Work out the finished part from the listing and answer in its coordinate system (mm). A direction names the side the tool comes from. Coordinates: 2 decimals unless noted, no trailing zeros. Order: outer loops, then holes, each group sorted by start corner. A loop starts at its lowest first (then second) coordinate and runs counter-clockwise, first axis right, second up. Notation, with made-up numbers: (33, 76.5) - (47, 76.5) arc R18 cw to (47, 80.5) - close; hole circle Ø10 at (47, 4.25). An arc over 180 degrees is marked (long way). Answer as a JSON object with one key per item and string values. Group by question number.
1) Find the intervals of material crossed by line 1 along Y through (x, z) = (17, 0) (3 decimals); line 2 along Y through (x, z) = (26.5, 0) (3 decimals); line 3 along Y through (x, z) = (-30, 9), in increasing order.
2) Each of these flat-tipped pins is pushed along its axis until it touches: P1, Ø4, axis at y = 21.5, z = 16.5, coming from the -X side; P2, Ø6, axis at x = 8.5, y = 18.5, coming from the -Z side; P3, Ø23, axis at x = 8.5, z = -17, coming from the +Y side. Where does it stop, or does it pass through?
3) Section D-D (y = 12.7) is taken. Give the vertices of the cut face in (x, z) (3 decimals).
4) Section B-B (x = 24) is taken. Give the vertices of the cut face in (y, z) (3 decimals).
5) Section C-C (y = 7) is taken. Give the vertices of the cut face in (x, z).
6) A tool of negligible diameter and unlimited length cuts with its end or side. For faces 1 (the face through (25, 30.48, 0)), 2 (the face through (21.37, 27.9, 3.09)), from which of +Z, -Z, +X, -X, +Y, -Y can it reach the whole face along a straight path? Write none if from no direction.
7) Section A-A (z = 0) is taken. Give the vertices of the cut face in (x, y) (3 decimals), plus the area to 3 significant figures.
from build123d import *

# Parameters (mm, degrees)
SKETCH1_R               = 38.1
BOSS_EXTRUDE1_DEPTH     = 25.4
SKETCH2_R               = 5.08
BOSS_EXTRUDE2_DEPTH     = 5.08
SKETCH3_R               = 1.905
CUT_EXTRUDE1_DEPTH      = 46.228
CUT_EXTRUDE1_DEPTH_BACK = 46.482


with BuildPart() as part:
    # Sketch1 → Boss-Extrude1 (new body)
    with BuildSketch(Plane(origin=(0, 0, 0), x_dir=(1, 0, 0), z_dir=(0, 1, 0))):
        Circle(SKETCH1_R)
    extrude(amount=BOSS_EXTRUDE1_DEPTH)

    # Sketch2 → Boss-Extrude2 (add)
    with BuildSketch(Plane(origin=(0, 25.4, 0), x_dir=(1, 0, 0), z_dir=(0, 1, 0))):
        with Locations((25.4, 0)):
            Circle(SKETCH2_R)
    extrude(amount=BOSS_EXTRUDE2_DEPTH)

    # Sketch3 → Cut-Extrude1 (cut, two sides)
    with BuildSketch(Plane(origin=(0, 0, 0), x_dir=(0, 0, -1), z_dir=(1, 0, 0))) as cut_extrude1_sk:
        with Locations((0, 12.7)):
            Circle(SKETCH3_R)
    extrude(amount=CUT_EXTRUDE1_DEPTH, mode=Mode.SUBTRACT)
    extrude(cut_extrude1_sk.sketch, amount=-CUT_EXTRUDE1_DEPTH_BACK, mode=Mode.SUBTRACT)


solid = part.part
Report:
{
 "1": {"line 1": "y = 0 to 10.795, 14.605 to 25.4", "line 2": "y = 0 to 10.795, 14.605 to 30.48", "line 3": "y = 0 to 25.4"},
 "2": {"P1": "stops at x = -35.23", "P2": "stops at z = -37.7", "P3": "stops at y = 25.4"},
 "3": {"outline": "(-38.052, -1.905) arc R38.1 ccw to (38.052, -1.905) - close; (-38.052, 1.905) - (38.052, 1.905) arc R38.1 ccw to start"},
 "4": {"outline": "(0, -29.591) - (25.4, -29.591) - (25.4, -4.883) - (30.48, -4.883) - (30.48, 4.883) - (25.4, 4.883) - (25.4, 29.591) - (0, 29.591) - close; hole circle Ø3.81 at (12.7, 0)"},
 "5": {"outline": "circle Ø76.2 at (0, 0)"},
 "6": {"face 1": "+Z, -Z, +X, -X, +Y", "face 2": "+Y"},
 "7": {"outline": "(-38.1, 0) - (38.1, 0) - (38.1, 10.795) - (-38.1, 10.795) - close; (-38.1, 14.605) - (38.1, 14.605) - (38.1, 25.4) - (30.48, 25.4) - (30.48, 30.48) - (20.32, 30.48) - (20.32, 25.4) - (-38.1, 25.4) - close", "area": "1,700 mm²"}
}
